```python
from build123d import *

# Parameters (mm, degrees)
F0_R     = 0.75
F0_W     = 3.175
F0_H     = 6
F1_DEPTH = 3.175


# Not quite as in the source:
# - a length typed as a fraction of an inch, garbled in the dataset ("3 / 203.2 mm" for 3/8 in), is restored


with BuildPart() as f1:
    # F0 (on Top) → F1 (new body)
    with BuildSketch(Plane.XY):
        Polygon((21.0674113333, 24.2020648569), (21.0674113333, 27.2020648569), (22.5674113333, 27.2020648569), (22.5674113333, 28.7020648569), (24.5674113333, 28.7020648569), (24.5674113333, 27.2020648569), (33.8924113333, 27.2020648569), (33.8924113333, 31.2020648569), (33.8924113333, 37.2020648569), (23.2424113333, 37.2020648569), (23.2424113333, 31.2020648569), (15.2424113333, 31.2020648569), (15.2424113333, 24.2020648569), (12.0674113333, 24.2020648569), (12.0674113333, 37.2020648569), (8.0674113333, 37.2020648569), (8.0674113333, 33.2020648569), (4.8924113333, 33.2020648569), (4.8924113333, 37.2020648569), (-21.7575886667, 37.2020648569), (-21.7575886667, 24.2020648569), (-24.9325886667, 24.2020648569), (-24.9325886667, 31.2020648569), (-32.9325886667, 31.2020648569), (-32.9325886667, 37.2020648569), (-38.7575886667, 37.2020648569), (-38.7575886667, 31.2020648569), (-38.7575886667, 27.2020648569), (-29.4325886667, 27.2020648569), (-29.4325886667, 28.7020648569), (-27.4325886667, 28.7020648569), (-27.4325886667, 27.2020648569), (-25.9325886667, 27.2020648569), (-25.9325886667, 24.2020648569), (-27.4325886667, 24.2020648569), (-27.4325886667, 22.7020648569), (-29.4325886667, 22.7020648569), (-29.4325886667, 24.2020648569), (-38.7575886667, 24.2020648569), (-38.7575886667, 20.2020648569), (-38.7575886667, 14.2020648569), (33.8924113333, 14.2020648569), (33.8924113333, 20.2020648569), (33.8924113333, 24.2020648569), (24.5674113333, 24.2020648569), (24.5674113333, 22.7020648569), (22.5674113333, 22.7020648569), (22.5674113333, 24.2020648569), align=None)
        with Locations((-17.1825886667, 20.2020648569)):
            Circle(F0_R, mode=Mode.SUBTRACT)
        with Locations((-6.1825886667, 20.2020648569)):
            Circle(F0_R, mode=Mode.SUBTRACT)
        with Locations((-17.1825886667, 31.2020648569)):
            Circle(F0_R, mode=Mode.SUBTRACT)
        with Locations((-6.1825886667, 31.2020648569)):
            Circle(F0_R, mode=Mode.SUBTRACT)
        with Locations((35.4799113333, 34.2020648569)):
            Rectangle(F0_W, F0_H)
        with Locations((35.4799113333, 17.2020648569)):
            Rectangle(F0_W, F0_H)
    extrude(amount=F1_DEPTH)


solid = f1.part
```
The model under review builds one solid part; all positions refer to its coordinate system, in mm. A direction names the side the tool comes from. Give positions to 0.01 mm unless a question says otherwise; leave off trailing zeros. Loops run counter-clockwise (first coordinate to the right, second up) from the corner with the lowest first, then second, coordinate; pieces in that order, holes last. Notation, with made-up numbers: (-5.5, 51.5) - (20.5, 51.5) arc R11 ccw to (20.5, 60.5) - close; hole circle Ø10 at (-4, 60). An arc over 180 degrees is marked (long way). Answer as a JSON object with one key per item and string values.
Q1. Mouldability with a two-part tool opening along Z and no side actions: class faces 5 (the flat face through (-1, 26, 0)), 6 (the flat face through (-36, 37.202, 2)) as +Z half, -Z half, draft (parallel to the pull), parting line (faces both ways), or undercut.
Worked out:
{"face 5": "-Z half", "face 6": "draft"}
Q2. Add section D-D on y = 22. State the section outline as (x, z) points (3 decimals).
Worked out:
{"outline": "(-38.758, 0) - (33.892, 0) - (33.892, 3.175) - (-38.758, 3.175) - close"}
Q3. For faces 1 (the flat face through (29, 24.202, 2)), 2 (the flat face through (-23, 24.202, 2)), 3 (the flat face through (-34, 24.202, 2)), 4 (the flat face through (-27.433, 28, 2)), list the 3-axis set-ups (+Z, -Z, +X, -X, +Y, -Y) from which the entire face can be reached by the end or side of a thin tool; tool diameter is ignored.
Worked out:
{"face 1": "+Z, -Z, +X", "face 2": "+Z, -Z, +Y", "face 3": "+Z, -Z, -X", "face 4": "+Z, -Z"}
Q4. To check wall thickness, follow line 1 along X through (y, z) = (30, 2.6); line 2 along X through (y, z) = (23.5, 0.7); line 3 along X through (y, z) = (34.25, 0.7). State the ranges of each line that lie inside material, in increasing order.
Worked out:
{"line 1": "x = -38.76 to -24.93, -21.76 to 12.07, 15.24 to 33.89", "line 2": "x = -38.76 to -29.43, -27.43 to 22.57, 24.57 to 33.89", "line 3": "x = -38.76 to -32.93, -21.76 to 4.89, 8.07 to 12.07, 23.24 to 37.07"}
Q5. Add section A-A on y = 26. State the section outline as (x, z) points (3 decimals).
Worked out:
{"outline": "(-25.933, 0) - (-24.933, 0) - (-24.933, 3.175) - (-25.933, 3.175) - close; (-21.758, 0) - (12.067, 0) - (12.067, 3.175) - (-21.758, 3.175) - close; (15.242, 0) - (21.067, 0) - (21.067, 3.175) - (15.242, 3.175) - close"}
Q6. Add section C-C on z = 2.65. Count the separate pieces of the cut face and the enclosed holes in it, plus the area to 3 significant figures.
Worked out:
{"separate pieces": "1", "enclosed holes": "4", "area": "1,420 mm^2"}
Q7. Add section B-B on x = 13.5. State the section outline as (y, z) points (3 decimals).
Worked out:
{"outline": "(14.202, 0) - (24.202, 0) - (24.202, 3.175) - (14.202, 3.175) - close"}
Q8. Insertion check: pin 1 (2 mm diameter, centred on x = -6.18, y = 31.2, fed in from -Z); pin 2 (1.4 mm diameter, centred on x = -6.18, y = 20.2, fed in from +Z); pin 3 (1.6 mm diameter, centred on x = 6.5, z = 1, fed in from +Y); pin 4 (0.8 mm diameter, centred on y = 23.5, z = 1.5, fed in from +X). Each pin has a flat end and moves straight along its axis. Give the tip position at first contact, or say it passes through.
Worked out:
{"pin 1": "stops at z = 0", "pin 2": "passes through", "pin 3": "stops at y = 33.2", "pin 4": "stops at x = 33.89"}
